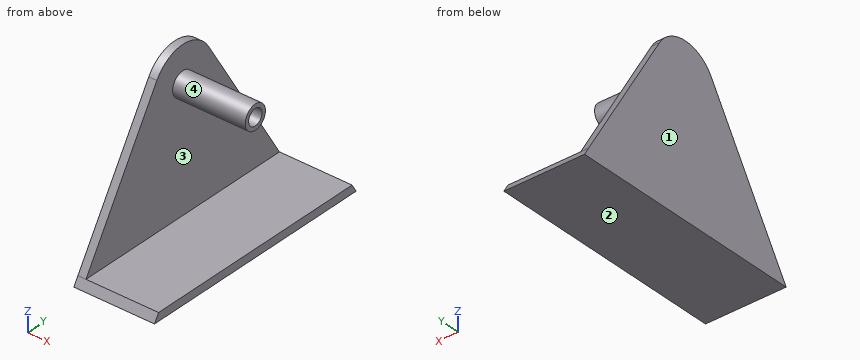
from build123d import *

# Parameters (mm, degrees)
F0_R     = 15
F1_DEPTH = 10
F0_R_2   = 10
F2_DEPTH = 100
F0_R_3   = 8
F3_DEPTH = 10
F4_DEPTH = 10
F5_DEPTH = 100


with BuildPart() as f1:
    # F0 (on Right) → F1 (new body)
    with BuildSketch(Plane.YZ):
        Polygon((-150, 0), (0, 0), (150, 0), (143.916984, 10), (0, 10), (-143.916984, 10), align=None)
        with BuildLine():
            Line((-38.445662, 183.386558), (-143.916984, 10))
            Line((-143.916984, 10), (0, 10))
            Line((0, 10), (143.916984, 10))
            Line((143.916984, 10), (38.445662, 183.386558))
            ThreePointArc((38.445662, 183.386558), (43.330444, 172.14383), (45, 160))
            ThreePointArc((45, 160), (-12.14383, 116.669556), (-38.445662, 183.386558))
        make_face()
        with BuildLine():
            ThreePointArc((38.445662, 183.386558), (0, 205), (-38.445662, 183.386558))
            ThreePointArc((-38.445662, 183.386558), (-12.14383, 116.669556), (45, 160))
            ThreePointArc((45, 160), (43.330444, 172.14383), (38.445662, 183.386558))
        make_face()
        with Locations((0, 160)):
            Circle(F0_R, mode=Mode.SUBTRACT)
    extrude(amount=F1_DEPTH)

    # F0 (on Right) → F2 (join)
    with BuildSketch(Plane.YZ):
        with Locations((0, 160)):
            Circle(F0_R)
        with Locations((0, 160)):
            Circle(F0_R_2, mode=Mode.SUBTRACT)
    extrude(amount=F2_DEPTH)

    # F0 (on Right) → F3 (join)
    with BuildSketch(Plane.YZ):
        with Locations((0, 160)):
            Circle(F0_R_2)
        with Locations((0, 160)):
            Circle(F0_R_3, mode=Mode.SUBTRACT)
    extrude(amount=F3_DEPTH)

    # F0 (on Right) → F4 (join)
    with BuildSketch(Plane.YZ):
        with Locations((0, 160)):
            Circle(F0_R_3)
    extrude(amount=F4_DEPTH)

    # F0 (on Right) → F5 (join)
    with BuildSketch(Plane.YZ):
        Polygon((-150, 0), (0, 0), (150, 0), (143.916984, 10), (0, 10), (-143.916984, 10), align=None)
    extrude(amount=F5_DEPTH)


solid = f1.part
Design review of the part built by this model. Coordinates are the model's own, in mm. Face numbers are marked on the shaded views. Give positions to 0.01 mm unless a question says otherwise; leave off trailing zeros. Loops run counter-clockwise (first coordinate to the right, second up) from the corner with the lowest first, then second, coordinate; pieces in that order, holes last. Notation, with made-up numbers: M 85,16 L 139,16 A23 cw 139,30 Z; hole C -26,6.5 d6. An arc over 180 degrees is marked long. Answer as a JSON object with one key per item and string values.
Item 1: We need section B-B (y = 0). State the section outline as (x, z) points.
Output values:
{"outline": "M 0,0 L 100,0 L 100,10 L 10,10 L 10,145 L 100,145 L 100,150 L 10,150 L 10,170 L 100,170 L 100,175 L 10,175 L 10,205 L 0,205 Z"}
Item 2: Wall thickness on line 1 along Z through (x, y) = (34.5, 0); line 2 along X through (y, z) = (-98.5, 37): over which ranges is each line inside the solid? List them lowest first.
Output values:
{"line 1": "z = 0 to 10, 145 to 150, 170 to 175", "line 2": "x = 0 to 10"}
Item 3: We need section D-D (y = 96.5). State the section outline as (x, z) points, and give its area (3 significant figures).
Output values:
{"outline": "M 0,0 L 100,0 L 100,10 L 10,10 L 10,87.95 L 0,87.95 Z", "area": "1,780 mm2"}
Item 4: Mouldability with a two-part tool opening along Z and no side actions: class the marked faces 1, 2, 3 and 4 as pulls with the +Z half, pulls with the -Z half, needs draft (parallel to the pull), parting line crosses it, or undercut.
Output values:
{"face 1": "needs draft", "face 2": "pulls with the -Z half", "face 3": "undercut", "face 4": "undercut"}
Item 5: We need section A-A (x = 14.5). State the section outline as (y, z) points.
Output values:
{"outline": "M -150,0 L 150,0 L 143.92,10 L -143.92,10 Z; C 0,160 d30; hole C 0,160 d20"}
Item 6: We need section C-C (z = 160). State the section outline as (x, y) points, and give its area (3 significant figures).
Output values:
{"outline": "M 0,-52.67 L 10,-52.67 L 10,-15 L 100,-15 L 100,-10 L 10,-10 L 10,10 L 100,10 L 100,15 L 10,15 L 10,52.67 L 0,52.67 Z", "area": "1,950 mm2"}
Item 7: For P1, Ø6, axis at y = 2.5, z = 156.5, coming from the +X side; P2, Ø1, axis at x = 70, y = 95, coming from the +Z side; P3, Ø2, axis at x = 63.5, z = 174.5, coming from the +Y side, all flat-tipped, find the tip position at first contact; note any pin that passes through.
Output values:
{"P1": "stops at x = 10", "P2": "stops at z = 10", "P3": "stops at y = 6.54"}
